The model under review builds one solid part; all positions refer to its coordinate system, in mm. A direction names the side the tool comes from. Round coordinates to 2 decimals unless told otherwise and drop trailing zeros. Order: outer loops, then holes, each group sorted by start corner. A loop starts at its lowest first (then second) coordinate and runs counter-clockwise, first axis right, second up. Notation, with made-up numbers: M 30.25,-37 L 86.25,-37 A25 ccw 86.25,-20 Z; hole C 17.25,73 d10. An arc over 180 degrees is marked long. One line per item, written item: value. Start each with the question number.
from build123d import *

# Parameters (mm, degrees)
BOX_W           = 180
BOX_H           = 140
BOX_DEPTH       = 6
SKETCH_W        = 180
SKETCH_H        = 140
PAD_DEPTH       = 60
SKETCH007_R     = 2.1
POCKET001_DEPTH = 35


with BuildPart() as part:
    # Box → Box (new body)
    with BuildSketch(Plane.XY):
        with Locations((90, 70)):
            Rectangle(BOX_W, BOX_H)
    extrude(amount=BOX_DEPTH)

    # Sketch → Pad (new body)
    with BuildSketch(Plane.XY.offset(6)):
        with Locations((90, 70)):
            Rectangle(SKETCH_W, SKETCH_H)
        Polygon((166.928932, 134), (13.071068, 134), (6, 126.928932), (6, 13.071068), (13.071068, 6), (166.928932, 6), (174, 13.071068), (174, 126.928932), align=None, mode=Mode.SUBTRACT)
    extrude(amount=PAD_DEPTH)

    # Sketch007 → Pocket001 (cut)
    with BuildSketch(Plane.XY.offset(66)):
        with Locations((172.285714, 6)):
            Circle(SKETCH007_R)
        with Locations((172.285714, 134)):
            Circle(SKETCH007_R)
        with Locations((7.714286, 134)):
            Circle(SKETCH007_R)
        with Locations((7.714286, 6)):
            Circle(SKETCH007_R)
    extrude(amount=-POCKET001_DEPTH, mode=Mode.SUBTRACT)


solid = part.part
Item 1: Machinability: for faces 4 (the cylindrical face through (174.226, 133.196, 48.745)), 5 (the flat face through (89, 0, 33)), which of the approach directions +Z, -Z, +X, -X, +Y, -Y give a long, thin tool a straight path to every point of the face, cutting with its end or side? Answer none if there is none.
Item 2: Consider section D-D, the plane x = 133. Give the boundary of the cut face in (y, z).
Item 3: The part is to be moulded in two halves that separate along X. For faces 1 (the flat face through (0, 69, 33)), 2 (the flat face through (89, 71, 0)), 3 (the flat face through (9.585, 130.514, 35.58)), say which applies: pulls with the +X half, pulls with the -X half, needs draft (parallel to the pull), parting line crosses it, or undercut.
Item 4: Wall thickness on L1, parallel to X at y = 65.5, z = 48; L2, parallel to Y at x = 37, z = 42; L3, parallel to Z at x = 85, y = 100: over which ranges is each line inside the solid? List them lowest first.
Item 5: Consider section B-B, the plane z = 13.5. Give the boundary of the cut face in (x, y), then the cut area to 3 significant figures.
Item 6: Consider section A-A, the plane z = 57. Give the boundary of the cut face in (x, y).
Item 7: Clearance check with flat-ended pins moving along their axes: P1, Ø1, axis at x = 160.5, y = 92, coming from the +Z side; P2, Ø3.5, axis at x = 172.29, y = 134, coming from the +Z side. State where each tip first meets the part, or that it passes through.
Item 8: Consider section C-C, the plane y = 94. Give the boundary of the cut face in (x, z).
Computed:
1. face 4: +Z
1. face 5: +Z, -Z, +X, -X, -Y
2. outline: M 0,0 L 140,0 L 140,66 L 134,66 L 134,6 L 6,6 L 6,66 L 0,66 Z
3. face 1: pulls with the -X half
3. face 2: needs draft
3. face 3: undercut
4. L1: x = 0 to 6, 174 to 180
4. L2: y = 0 to 6, 134 to 140
4. L3: z = 0 to 6
5. outline: M 0,0 L 180,0 L 180,140 L 0,140 Z; hole M 6,13.07 L 13.07,6 L 166.93,6 L 174,13.07 L 174,126.93 L 166.93,134 L 13.07,134 L 6,126.93 Z
5. area: 3,800 mm^2
6. outline: M 0,0 L 180,0 L 180,140 L 0,140 Z; hole C 7.71,6 d4.2; hole C 7.71,134 d4.2; hole M 6,13.07 L 13.07,6 L 166.93,6 L 174,13.07 L 174,126.93 L 166.93,134 L 13.07,134 L 6,126.93 Z; hole C 172.29,6 d4.2; hole C 172.29,134 d4.2
7. P1: stops at z = 6
7. P2: stops at z = 31
8. outline: M 0,0 L 180,0 L 180,66 L 174,66 L 174,6 L 6,6 L 6,66 L 0,66 Z
